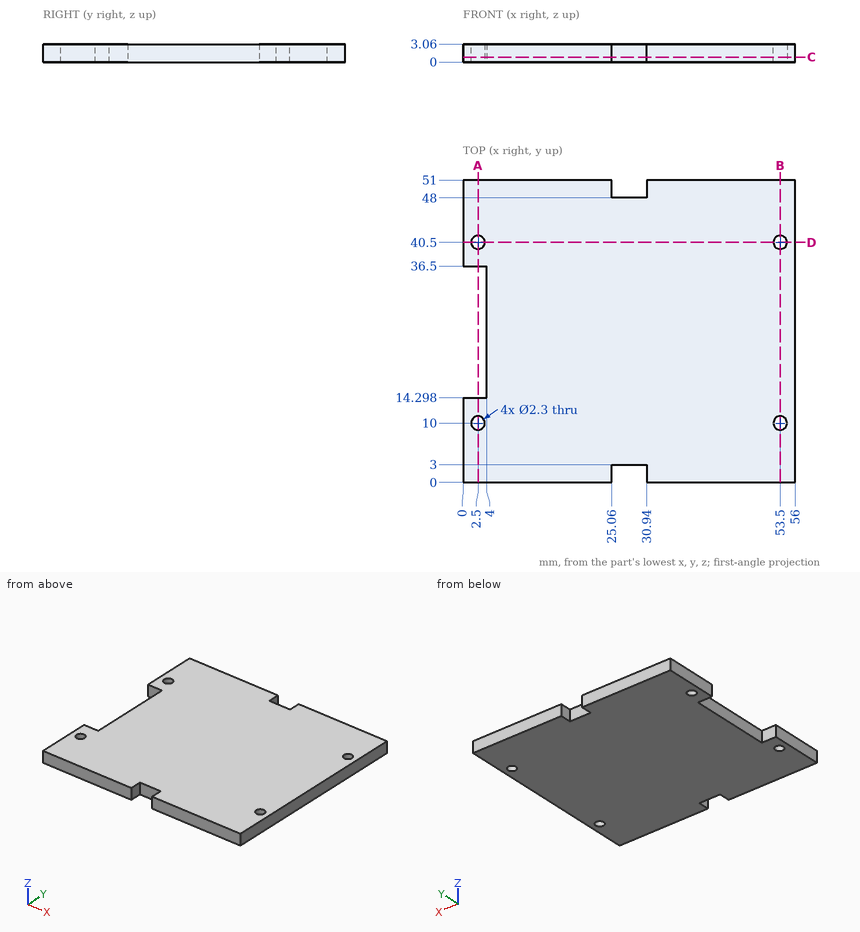
Input: dimensioned drawing with shaded views. Units: mm. Origin: part minimum x, y, z. Give positions to 0.01 mm unless a question says otherwise; leave off trailing zeros. Write each loop counter-clockwise with the first axis right and the second up, starting at its lowest first coordinate (ties: lowest second). Pieces come first, ordered by that corner, then holes. Notation, with made-up numbers: M 75.25,86.5 L 94.25,86.5 A21 cw 94.25,109.5 Z; hole C -20,28 d1. An arc over 180 degrees is marked long. Write item = value, one per line. Start each with the question number.
1) Cut plane B-B on x = 53.5. Return the cut outline in (y, z).
2) Cut plane D-D on y = 40.5. Return the cut outline in (x, z), then the cut area to 3 significant figures.
3) Material intervals for line 1 along Y through (x, z) = (2.5, 1.3); line 2 along Y through (x, z) = (3, 0.8); line 3 along X through (y, z) = (19, 2.3), sorted ascending. Write a range as [from, to].
4) Cut plane C-C on z = 0.85. Return the cut outline in (x, y).
5) First-contact query: pin 1 Ø0.9 at (x, z) = (28.5, 2) entering from -Y; pin 2 Ø6 at (x, y) = (7.5, 45.5) entering from -Z; pin 3 Ø1.5 at (y, z) = (27.5, 2) entering from -X. Flat tips, straight axial feed; report the tip coordinate or a pass-through.
6) Cut plane A-A on x = 2.5. Return the cut outline in (y, z).
Solved:
q1.outline = M 0,0 L 8.85,0 L 8.85,3.06 L 0,3.06 Z; M 11.15,0 L 39.35,0 L 39.35,3.06 L 11.15,3.06 Z; M 41.65,0 L 51,0 L 51,3.06 L 41.65,3.06 Z
q2.outline = M 0,0 L 1.35,0 L 1.35,3.06 L 0,3.06 Z; M 3.65,0 L 52.35,0 L 52.35,3.06 L 3.65,3.06 Z; M 54.65,0 L 56,0 L 56,3.06 L 54.65,3.06 Z
q2.area = 157 mm2
q3.line_1 = [0, 8.85], [11.15, 14.3], [36.5, 39.35], [41.65, 51]
q3.line_2 = [0, 8.96], [11.04, 14.3], [36.5, 39.46], [41.54, 51]
q3.line_3 = [4, 56]
q4.outline = M 0,0 L 25.06,0 L 25.06,3 L 30.94,3 L 30.94,0 L 56,0 L 56,51 L 30.94,51 L 30.94,48 L 25.06,48 L 25.06,51 L 0,51 L 0,36.5 L 4,36.5 L 4,14.3 L 0,14.3 Z; hole C 2.5,10 d2.3; hole C 2.5,40.5 d2.3; hole C 53.5,10 d2.3; hole C 53.5,40.5 d2.3
q5.pin_1 = 3
q5.pin_2 = 0
q5.pin_3 = 4
q6.outline = M 0,0 L 8.85,0 L 8.85,3.06 L 0,3.06 Z; M 11.15,0 L 14.3,0 L 14.3,3.06 L 11.15,3.06 Z; M 36.5,0 L 39.35,0 L 39.35,3.06 L 36.5,3.06 Z; M 41.65,0 L 51,0 L 51,3.06 L 41.65,3.06 Z
